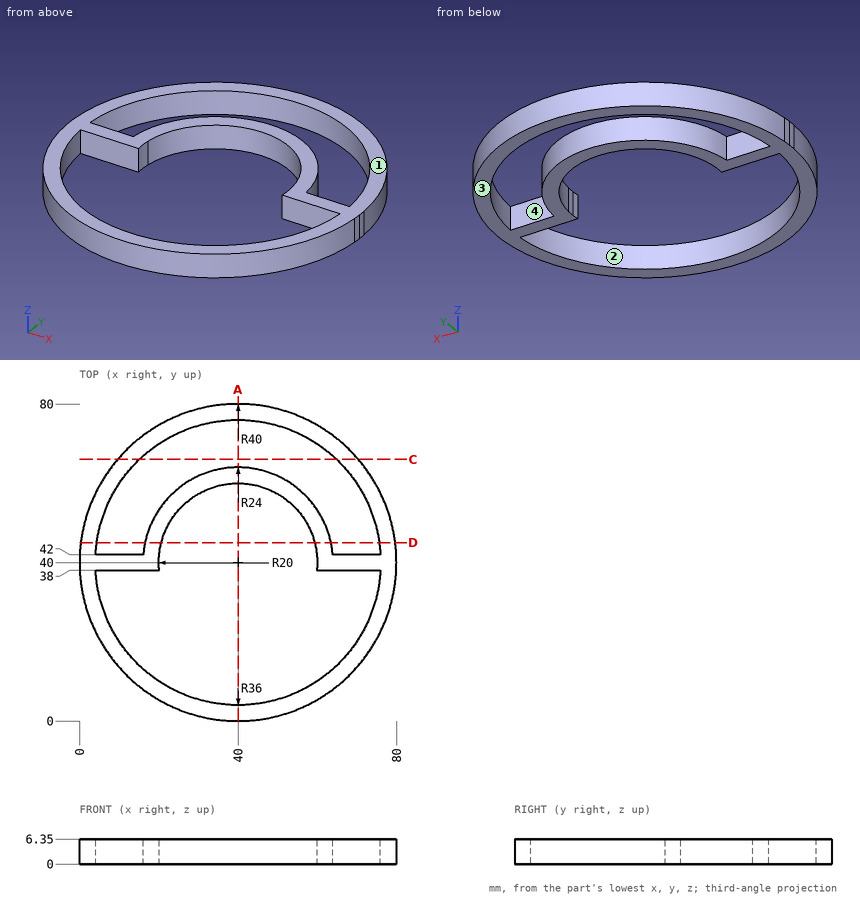
Check sheet for the drawn part. Datum: minimum x, y, z corner. Units: mm. A direction names the side the tool comes from. Give positions to 0.01 mm unless a question says otherwise; leave off trailing zeros. Loops run counter-clockwise (first coordinate to the right, second up) from the corner with the lowest first, then second, coordinate; pieces in that order, holes last. Notation, with made-up numbers: M 31,52.25 L 85,52.25 A33 ccw 85,83.25 Z; hole C 55.5,72.25 d11. An arc over 180 degrees is marked long. Return JSON: item names as keys, results as strings.
1) Section check C-C, the plane y = 66. Enter the section's corners in (x, z), and give its area (3 significant figures).
Findings:
{"outline": "M 9.6,0 L 15.1,0 L 15.1,6.35 L 9.6,6.35 Z; M 64.9,0 L 70.4,0 L 70.4,6.35 L 64.9,6.35 Z", "area": "69.8 mm2"}
2) Material ranges on L1, parallel to Y at x = 24, z = 5.5; L2, parallel to Y at x = 10.5, z = 5; L3, parallel to X at y = 53, z = 5.5, recorded low to high. Write a range as [from, to].
Findings:
{"L1": "y = [3.34, 7.75], [52, 57.89], [72.25, 76.66]", "L2": "y = [12.99, 19.37], [38, 42], [60.63, 67.01]", "L3": "x = [2.17, 6.43], [19.83, 24.8], [55.2, 60.17], [73.57, 77.83]"}
3) Section check A-A, the plane x = 40. Enter the section's corners in (y, z).
Findings:
{"outline": "M 0,0 L 4,0 L 4,6.35 L 0,6.35 Z; M 60,0 L 64,0 L 64,6.35 L 60,6.35 Z; M 76,0 L 80,0 L 80,6.35 L 76,6.35 Z"}
4) Gauge pin test, flat ends, axial feed: P1, Ø1.9, axis at x = 8, z = 3.5, coming from the -Y side; P2, Ø1, axis at y = 19, z = 5, coming from the +X side; P3, Ø1.5, axis at y = 71, z = 3, coming from the -X side. Record the tip position at first contact, or that the pin passes through.
Findings:
{"P1": "stops at y = 14.78", "P2": "stops at x = 74.35", "P3": "stops at x = 13.83"}
5) Section check D-D, the plane y = 45. Enter the section's corners in (x, z).
Findings:
{"outline": "M 0.31,0 L 4.35,0 L 4.35,6.35 L 0.31,6.35 Z; M 16.53,0 L 20.64,0 L 20.64,6.35 L 16.53,6.35 Z; M 59.36,0 L 63.47,0 L 63.47,6.35 L 59.36,6.35 Z; M 75.65,0 L 79.69,0 L 79.69,6.35 L 75.65,6.35 Z"}
6) Tool access check on the marked faces 3 and 4. Record the directions out of +Z, -Z, +X, -X, +Y, -Y that give a thin tool (end or side, any length) a straight path to the whole face; none if there is none.
Findings:
{"face 3": "-Z, +X, -X, +Y, -Y", "face 4": "+Z, -Z"}
7) Mould release check, pull along X, two halves, no side actions. Record for the marked faces 1 and 2: released by +X, released by -X, zero draft, split by the parting line, or undercut.
Findings:
{"face 1": "zero draft", "face 2": "undercut"}
